Autodesk Fusion 360 part; units mm, degrees
sketch "Sketch1" plane through (0, 0, 0) normal (0, 0, 1) x (1, 0, 0)
  line L0 (0, 0) -> (152.4, 0)
  line L1 (152.4, 0) -> (152.4, 127)
  line L2 (152.4, 127) -> (0, 127)
  line L3 (0, 127) -> (0, 0)
  line L4 (46.99, 109.22) -> (144.399, 109.22)
  line L5 (144.399, 109.22) -> (144.399, 17.78)
  line L6 (144.399, 17.78) -> (46.99, 17.78)
  line L7 (46.99, 17.78) -> (46.99, 109.22)
  dimension "d1" = 152.4
  dimension "d2" = 127
  dimension "d3" = 97.409
  dimension "d4" = 91.44
  dimension "d5" = 46.99
  dimension "d6" = 17.78
extrude "Extrude1" add sketch "Sketch1" along normal blind 2.54 contours L0 L1 L2 L3 | L4 L5 L6 L7
extrude "Extrude2" add sketch "Sketch1" along normal blind 5.715 contours L4 L5 L6 L7
sketch "Sketch2" plane through (0, 0, 5.715) normal (0, 0, 1) x (-1, 0, 0)
  line L0 (-46.99, -17.78) -> (-144.399, -17.78)
  line L1 (-144.399, -17.78) -> (-144.399, -109.22)
  line L2 (-144.399, -109.22) -> (-46.99, -109.22)
  line L3 (-46.99, -109.22) -> (-46.99, -17.78)
  line L4 (-46.99, -91.44) -> (-97.79, -91.44)
  line L5 (-97.79, -91.44) -> (-97.79, -30.48)
  line L6 (-97.79, -30.48) -> (-46.99, -30.48)
  line L7 (-46.99, -25.4) -> (-46.99, -30.48)
  line L8 (-46.99, -91.44) -> (-44.45, -91.44)
  line L9 (-44.45, -91.44) -> (-44.45, -30.48)
  line L10 (-44.45, -30.48) -> (-46.99, -30.48)
  line L11 (-46.99, -30.48) -> (-46.99, -91.44)
  dimension "d11" = 60.96
  dimension "d12" = 17.78
  dimension "d15" = 50.8
  dimension "d19" = 2.54
  dimension "d20" = 60.96
extrude "Extrude3" cut sketch "Sketch2" against normal blind 38.1 contours L3 L4 L5 L6 L11
extrude "Extrude4" cut sketch "Sketch2" against normal blind 60.96 contours L3 L8 L9 L10 L11
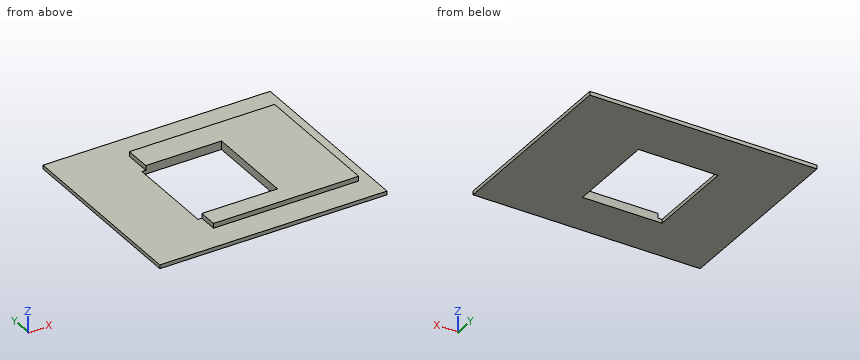
Here's how the part is built. I have some questions about the finished solid (model axes, mm). Round coordinates to 2 decimals unless told otherwise and drop trailing zeros. Order: outer loops, then holes, each group sorted by start corner. A loop starts at its lowest first (then second) coordinate and runs counter-clockwise, first axis right, second up. Notation, with made-up numbers: M 4.25,-6 L 25.25,-6 A4 cw 25.25,1 Z; hole C -20,-23.75 d5. An arc over 180 degrees is marked long. Return JSON: item names as keys, results as strings. Group by question number.
1. I'm going to push flat-ended pins straight in: pin 1 Ø1.6 at (y, z) = (97, 4) entering from -X; pin 2 Ø1.6 at (y, z) = (84, 3.5) entering from +X; pin 3 Ø1.6 at (x, z) = (108.5, 3.5) entering from -Y. Where does each tip first touch, or does it pass through?
2. If we section it at B-B on y = 39: List the corners of the cut face in (x, z) for me (3 decimals).
3. If we section it at C-C on x = 65: List the corners of the cut face in (y, z) for me (3 decimals).
4. Please list where these lines run through material, in increasing order: probe 1 along Y at (x, z) = (88.5, 1.65); probe 2 along X at (y, z) = (38.5, 1.4); probe 3 along Y at (x, z) = (97, 4.05).
5. If we section it at D-D on x = 126: List the corners of the cut face in (y, z) for me (3 decimals), then the cut area to 3 significant figures.
6. If we section it at A-A on z = 1.65: List the corners of the cut face in (x, y) for me, then the cut area to 3 significant figures.
Reply:
{
 "1": {"pin 1": "x = 46.99", "pin 2": "x = 144.4", "pin 3": "y = 17.78"},
 "2": {"outline": "M 0,0 L 44.45,0 L 44.45,2.54 L 0,2.54 Z; M 97.79,0 L 152.4,0 L 152.4,2.54 L 144.399,2.54 L 144.399,5.715 L 97.79,5.715 Z"},
 "3": {"outline": "M 0,0 L 30.48,0 L 30.48,5.715 L 17.78,5.715 L 17.78,2.54 L 0,2.54 Z; M 91.44,0 L 127,0 L 127,2.54 L 109.22,2.54 L 109.22,5.715 L 91.44,5.715 Z"},
 "4": {"probe 1": "0 to 30.48, 91.44 to 127", "probe 2": "0 to 44.45, 97.79 to 152.4", "probe 3": "17.78 to 30.48, 91.44 to 109.22"},
 "5": {"outline": "M 0,0 L 127,0 L 127,2.54 L 109.22,2.54 L 109.22,5.715 L 17.78,5.715 L 17.78,2.54 L 0,2.54 Z", "area": "613 mm^2"},
 "6": {"outline": "M 0,0 L 152.4,0 L 152.4,127 L 0,127 Z; hole M 44.45,30.48 L 97.79,30.48 L 97.79,91.44 L 44.45,91.44 Z", "area": "16,100 mm^2"}
}
